Can you work these out from the model? Positions are in its coordinate system, mm. A direction names the side the tool comes from. Round coordinates to 2 decimals unless told otherwise and drop trailing zeros. Write each loop counter-clockwise with the first axis right and the second up, starting at its lowest first coordinate (ties: lowest second). Pieces come first, ordered by that corner, then holes. Notation, with made-up numbers: (-36, 32) -> (7, 32) arc R13 cw to (7, 41) -> close; hole circle Ø5 at (77, 56.5). An arc over 180 degrees is marked (long way). Write item = value, one per line. Start each with the question number.
1) I'm going to push a flat-ended pin straight in: pin 1 (3 mm diameter, centred on x = 56.5, y = -4, fed in from -Z). Where does the tip first touch, or does it pass through?
2) Imagine slicing it at A-A, the plane y = -4. Please give me the cut outline in (x, z).
3) Imagine slicing it at C-C, the plane y = -11.5. Please give me the cut outline in (x, z), then the cut area to 3 significant figures.
4) Thinking about a two-plate mould opening in X: for faces 1 (the face through (37.025, -11.534, -3.042)), 2 (the face through (59.503, -8, -3)), 3 (the face through (55, -16, -3)), which applies, +X half, -X half, draft (parallel to the pull), parting line (faces both ways), or undercut?
5) If I drill on line 1 (Y direction, x = 38.5, z = -2.5); line 2 (X direction, y = -10.8, z = -4.45); line 3 (X direction, y = -11, z = -3.1), over which ranges is the centre line in solid material (lowest first)?
6) For faces 4 (the face through (51.391, -15, -3)), 5 (the face through (40, -16, -3)), which set-ups out of +Z, -Z, +X, -X, +Y, -Y let a thin tool reach every point of the face, with its end or its side?
7) Imagine slicing it at D-D, the plane x = 47.5. Please give me the cut outline in (y, z) (3 decimals).
8) Imagine slicing it at B-B, the plane z = -5.25. Please give me the cut outline in (x, y) (3 decimals).
from build123d import *

# Parameters (mm, degrees)
SZKIC1_W                    = 24
SZKIC1_H                    = 16
DODANIE_WYCI_GNI_CIE1_DEPTH = 6
WYTNIJ_WYCI_GNI_CIE1_DEPTH  = 6
SZKIC3_R                    = 1.55
WYTNIJ_WYCI_GNI_CIE2_DEPTH  = 62.908035593


with BuildPart() as part:
    # Szkic1 → Dodanie-wyciągnięcie1 (new body)
    with BuildSketch(Plane.XY):
        with Locations((47.502982034, -8)):
            Rectangle(SZKIC1_W, SZKIC1_H)
    extrude(amount=-DODANIE_WYCI_GNI_CIE1_DEPTH)

    # Szkic2 → Wytnij-wyciągnięcie1 (cut)
    with BuildSketch(Plane.XY.offset(-6)):
        with BuildLine():
            Line((43.614537615, -16), (43.614537615, -14.730541148))
            Line((43.614537615, -14.730541148), (43.186780246, -15.145805693))
            ThreePointArc((43.186780246, -15.145805693), (43.13517548, -15.093936528), (43.084193998, -15.041454619))
            ThreePointArc((43.084193998, -15.041454619), (47.502982034, -4.675), (51.921770071, -15.041454619))
            ThreePointArc((51.921770071, -15.041454619), (51.867648174, -15.097128633), (51.812824874, -15.152112096))
            Line((51.812824874, -15.152112096), (51.391426454, -14.730541148))
            Line((51.391426454, -14.730541148), (51.391426454, -16))
            Line((51.391426454, -16), (43.614537615, -16))
        make_face()
    extrude(amount=WYTNIJ_WYCI_GNI_CIE1_DEPTH, mode=Mode.SUBTRACT)

    # Szkic3 → Wytnij-wyciągnięcie2 (cut, through all)
    with BuildSketch(Plane(origin=(0, 0, -6), x_dir=(-1, 0, 0), z_dir=(0, 0, -1))):
        with Locations((-56.502982034, -12)):
            Circle(SZKIC3_R)
        with Locations((-56.502982034, -4)):
            Circle(SZKIC3_R)
        with Locations((-38.502982034, -4)):
            Circle(SZKIC3_R)
        with Locations((-38.502982034, -12)):
            Circle(SZKIC3_R)
    extrude(amount=-WYTNIJ_WYCI_GNI_CIE2_DEPTH, mode=Mode.SUBTRACT)


solid = part.part
Reported:
q1.pin_1 = through
q2.outline = (35.5, -6) -> (36.95, -6) -> (36.95, 0) -> (35.5, 0) -> close; (40.05, -6) -> (54.95, -6) -> (54.95, 0) -> (40.05, 0) -> close; (58.05, -6) -> (59.5, -6) -> (59.5, 0) -> (58.05, 0) -> close
q3.outline = (35.5, -6) -> (37.04, -6) -> (37.04, 0) -> (35.5, 0) -> close; (39.97, -6) -> (41.42, -6) -> (41.42, 0) -> (39.97, 0) -> close; (53.59, -6) -> (55.04, -6) -> (55.04, 0) -> (53.59, 0) -> close; (57.97, -6) -> (59.5, -6) -> (59.5, 0) -> (57.97, 0) -> close
q3.area = 35.8 mm²
q4.face_1 = undercut
q4.face_2 = +X half
q4.face_3 = draft
q5.line_1 = -16 to -13.55, -10.45 to -5.55, -2.45 to 0
q5.line_2 = 35.5 to 37.52, 39.48 to 41.38, 53.63 to 55.52, 57.48 to 59.5
q5.line_3 = 35.5 to 37.32, 39.69 to 41.38, 53.62 to 55.32, 57.69 to 59.5
q6.face_4 = +Z, -Z, -Y
q6.face_5 = +Z, -Z, +X, -X, -Y
q7.outline = (-4.675, -6) -> (0, -6) -> (0, 0) -> (-4.675, 0) -> close
q8.outline = (35.503, -16) -> (43.615, -16) -> (43.615, -14.731) -> (43.187, -15.146) arc R6.125 cw to (43.084, -15.041) arc R6.125 cw (long way) to (51.813, -15.152) -> (51.391, -14.731) -> (51.391, -16) -> (59.503, -16) -> (59.503, 0) -> (35.503, 0) -> close; hole circle Ø3.1 at (38.503, -12); hole circle Ø3.1 at (38.503, -4); hole circle Ø3.1 at (56.503, -12); hole circle Ø3.1 at (56.503, -4)
